Check sheet for the modelled part. Datum: model origin and axes. Units: mm. Face numbers are marked on the shaded views. A direction names the side the tool comes from. Coordinates: 2 decimals unless noted, no trailing zeros. Order: outer loops, then holes, each group sorted by start corner. A loop starts at its lowest first (then second) coordinate and runs counter-clockwise, first axis right, second up. Notation, with made-up numbers: M -16.5,64.5 L 2.5,64.5 A21 cw 2.5,82.5 Z; hole C -2.75,57 d6. An arc over 180 degrees is marked long. Answer in a Markdown table with one row per item. Add a question column.
from build123d import *

# Parameters (mm, degrees)
F1_DEPTH       = 35
F3_D           = 5
F3_START       = 1.7550021
F3_START_2     = 1.8205079
F3_CBORE_D     = 10
F3_CBORE_DEPTH = 8
F4_W           = 22.4
F4_H           = 2
F5_DEPTH       = 25
F6_R           = 6
F7_DEPTH       = 8


with BuildPart() as f1:
    # F0 (on Top) → F1 (new body, symmetric)
    with BuildSketch(Plane.XY):
        with BuildLine():
            ThreePointArc((-17.3192642082, 2.5086026559), (17.5, 0), (-17.3192642082, -2.5086026559))
            Line((-17.3192642082, -2.5086026559), (-28.1192642082, -2.5086026559))
            Line((-28.1192642082, -2.5086026559), (-28.1192642082, -10.9086026559))
            ThreePointArc((-28.1192642082, -10.9086026559), (-25.7761184577, -16.5654569054), (-20.1192642082, -18.9086026559))
            Line((-20.1192642082, -18.9086026559), (-7.9192642082, -18.9086026559))
            ThreePointArc((-7.9192642082, -18.9086026559), (20.5, 0), (-7.9192642082, 18.9086026559))
            Line((-7.9192642082, 18.9086026559), (-20.1192642082, 18.9086026559))
            ThreePointArc((-20.1192642082, 18.9086026559), (-25.7761184577, 16.5654569054), (-28.1192642082, 10.9086026559))
            Line((-28.1192642082, 10.9086026559), (-28.1192642082, 2.5086026559))
            Line((-28.1192642082, 2.5086026559), (-17.3192642082, 2.5086026559))
        make_face()
    extrude(amount=F1_DEPTH, both=True)

    # F3 (through all)
    # its depths count from where the whole tool has entered the part; down to there all is cleared
    with Locations(Plane.XZ.offset(18.9086026559)):
        with Locations((-20.1192642082, -24.25, -F3_START), (-20.1192642082, -9.25, -F3_START), (-20.1192642082, 9.25, -F3_START), (-20.2, 24.25, -F3_START_2)):
            CounterBoreHole(F3_D / 2, F3_CBORE_D / 2, F3_CBORE_DEPTH)

    # F4 (on Front) → F5 (cut, symmetric)
    with BuildSketch(Plane.XZ):
        with Locations((-16.9192642082, 0)):
            Rectangle(F4_W, F4_H)
    extrude(amount=F5_DEPTH, both=True, mode=Mode.SUBTRACT)

    # F6 (on face) → F7 (cut)
    with BuildSketch(Plane.XY.offset(35)):
        with Locations((0, -25)):
            Circle(F6_R)
        with Locations((17.6776695297, -17.6776695297)):
            Circle(F6_R)
        with Locations((25, 0)):
            Circle(F6_R)
        with Locations((17.6776695297, 17.6776695297)):
            Circle(F6_R)
        with Locations((0, 25)):
            Circle(F6_R)
    extrude(amount=-F7_DEPTH, mode=Mode.SUBTRACT)


solid = f1.part
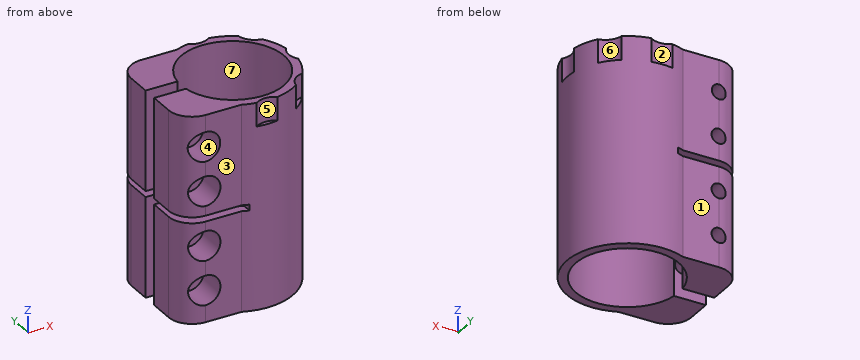
1. Section check D-D on x = -11. Enter the section's corners in (y, z).
2. Scan lines: line 1 (Z direction, x = -12.5, y = -13.5); line 2 (Z direction, x = -19.5, y = -5); line 3 (X direction, y = -6, z = 9). Record each from-to range of solid material in increasing order.
3. Section check B-B on x = 13. Enter the section's corners in (y, z), then the cut area to 3 significant figures.
4. Release check for a two-part mould opening along Y. For the marked faces 4, 5, 6 and 7 record: released by +Y, released by -Y, zero draft, split by the parting line, or undercut.
5. Go/stop test with flat-tipped pins: pin 1 Ø10 at (x, y) = (7.5, -6) entering from +Z; pin 2 Ø6 at (x, z) = (-20.2, 24.25) entering from +Y; pin 3 Ø8 at (y, z) = (-15, -27.5) entering from +X; pin 4 Ø3 at (x, z) = (-21, 11) entering from -Y. Record where each tip stops, or that it passes through.
6. Set-up check for the marked faces 1, 2 and 3: record each of +Z, -Z, +X, -X, +Y, -Y from which the full face is reachable in a straight line by a thin tool's end or side.
7. Section check C-C on z = 9.25. Enter the section's corners in (x, y), then the cut area to 3 significant figures.
8. Section check A-A on y = 5. Enter the section's corners in (x, z), then the cut area to 3 significant figures.
Result sheet:
| question | item | result |
|---|---|---|
| 1 | outline | M -18.91,-35 L -13.61,-35 L -13.61,-1 L -18.91,-1 Z; M -18.91,1 L -13.61,1 L -13.61,35 L -18.91,35 Z; M 13.61,-35 L 18.91,-35 L 18.91,-1 L 13.61,-1 Z; M 13.61,1 L 18.91,1 L 18.91,35 L 13.61,35 Z |
| 2 | line 1 | -35 to -1, 1 to 35 |
| 2 | line 2 | -35 to -26.67, -21.83 to -11.67, -6.83 to -1, 1 to 6.83, 11.67 to 21.85, 26.65 to 35 |
| 2 | line 3 | -28.12 to -22.61, -17.63 to -16.44, 16.44 to 19.6 |
| 3 | outline | M -15.85,-35 L -11.72,-35 L -11.72,35 L -13.92,35 L -13.92,27 L -15.85,27 Z; M 11.72,-35 L 15.85,-35 L 15.85,27 L 13.92,27 L 13.92,35 L 11.72,35 Z |
| 3 | area | 548 mm^2 |
| 4 | face 4 | zero draft |
| 4 | face 5 | released by -Y |
| 4 | face 6 | released by +Y |
| 4 | face 7 | undercut |
| 5 | pin 1 | through |
| 5 | pin 2 | y = 18.91 |
| 5 | pin 3 | x = 17.3 |
| 5 | pin 4 | y = -9.15 |
| 6 | face 1 | +Z, -Z, -X, +Y |
| 6 | face 2 | +Z, +Y |
| 6 | face 3 | +Z, -Z, -X, -Y |
| 7 | outline | M -28.12,-10.91 A8 ccw -25.12,-17.15 L -25.12,-9.15 L -22.62,-9.15 L -22.62,-2.51 L -28.12,-2.51 Z; M -28.12,2.51 L -22.62,2.51 L -22.62,18.51 A8 ccw -28.12,10.91 Z; M -17.62,-9.15 L -15.12,-9.15 L -15.12,-18.91 L -7.92,-18.91 A20.5 ccw long -7.92,18.91 L -17.62,18.91 L -17.62,2.51 L -17.32,2.51 A17.5 cw long -17.32,-2.51 L -17.62,-2.51 Z |
| 7 | area | 488 mm^2 |
| 8 | outline | M -28.12,-35 L -16.77,-35 L -16.77,-1 L -28.12,-1 Z; M -28.12,1 L -16.77,1 L -16.77,35 L -28.12,35 Z; M 16.77,-35 L 19.88,-35 L 19.88,35 L 16.77,35 Z; hole C -20.2,24.25 d5; hole C -20.12,-24.25 d5; hole C -20.12,-9.25 d5; hole C -20.12,9.25 d5 |
| 8 | area | 911 mm^2 |
